from build123d import *
from build123d.topology import SkipClean

# Parameters (mm, degrees)
SKETCH1_W                  = 22
SKETCH1_H                  = 39
SKETCH1_W_2                = 6
SKETCH1_H_2                = 8
BOSS_EXTRUDE1_DEPTH        = 8.25
SKETCH8_W                  = 15.1
SKETCH8_H                  = 11.4
CUT_EXTRUDE3_DEPTH         = 2.25
SKETCH7_R                  = 2.825
SKETCH7_R_2                = 0.825
CUT_EXTRUDE4_DEPTH         = 1.25
SKETCH9_R                  = 0.75
CUT_EXTRUDE5_DEPTH         = 39.274404999
CUT_EXTRUDE1_DEPTH         = 37.440988331
CUT_EXTRUDE1_DEPTH_BACK    = 39.690988331
CUT_EXTRUDE1_START         = 2.25
SKETCH6_R                  = 2.825
BOSS_EXTRUDE2_DEPTH        = 8.25
FILLET3_R                  = 4
FILLET4_R                  = 2
CUT_EXTRUDE7_DEPTH         = 39.900472274
FILLET5_R                  = 7
F_2_2_2_2_DIAMETER_HOLE1_D = 2.2
FILLET6_R                  = 2


with BuildPart() as part:
    # Sketch1 → Boss-Extrude1 (new body)
    with BuildSketch(Plane(origin=(0, 0, 0), x_dir=(1, 0, 0), z_dir=(0, 1, 0))):
        with Locations((21.383330249, 0)):
            Rectangle(SKETCH1_W, SKETCH1_H)
        with Locations((22.383330249, 0)):
            Rectangle(SKETCH1_W_2, SKETCH1_H_2, mode=Mode.SUBTRACT)
    extrude(amount=BOSS_EXTRUDE1_DEPTH)

    # Sketch8 → Cut-Extrude3 (cut)
    with BuildSketch(Plane(origin=(0, 8.25, 0), x_dir=(1, 0, 0), z_dir=(0, 1, 0))):
        with Locations((23.333330249, -12)):
            Rectangle(SKETCH8_W, SKETCH8_H)
        with Locations((23.333330249, 12)):
            Rectangle(SKETCH8_W, SKETCH8_H)
    extrude(amount=-CUT_EXTRUDE3_DEPTH, mode=Mode.SUBTRACT)

    # Sketch7 → Cut-Extrude4 (cut)
    with BuildSketch(Plane(origin=(0, 6, 0), x_dir=(1, 0, 0), z_dir=(0, 1, 0))):
        with Locations(Location((24.633330249, 12, 0), (0, 0, 270))):
            Circle(SKETCH7_R)
        with Locations(Location((20.140330249, 14.5, 0), (0, 0, 270))):
            Circle(SKETCH7_R_2)
        with Locations(Location((27.633330249, 14.5, 0), (0, 0, 270))):
            Circle(SKETCH7_R_2)
        with Locations(Location((27.633330249, 9.5, 0), (0, 0, 270))):
            Circle(SKETCH7_R_2)
        with Locations(Location((20.140330249, 9.5, 0), (0, 0, 270))):
            Circle(SKETCH7_R_2)
        with Locations(Location((20.140330249, -9.5, 0), (0, 0, 90))):
            Circle(SKETCH7_R_2)
        with Locations(Location((27.633330249, -9.5, 0), (0, 0, 90))):
            Circle(SKETCH7_R_2)
        with Locations(Location((27.633330249, -14.5, 0), (0, 0, 90))):
            Circle(SKETCH7_R_2)
        with Locations(Location((20.140330249, -14.5, 0), (0, 0, 90))):
            Circle(SKETCH7_R_2)
        with Locations(Location((24.633330249, -12, 0), (0, 0, 90))):
            Circle(SKETCH7_R)
    extrude(amount=-CUT_EXTRUDE4_DEPTH, mode=Mode.SUBTRACT)

    # Sketch9 → Cut-Extrude5 (cut, through all)
    with BuildSketch(Plane(origin=(0, 6, 0), x_dir=(1, 0, 0), z_dir=(0, 1, 0))):
        with Locations(Location((17.633330249, 14.5, 0), (0, 0, 270))):
            Circle(SKETCH9_R)
        with Locations(Location((17.633330249, 12, 0), (0, 0, 270))):
            Circle(SKETCH9_R)
        with Locations(Location((17.633330249, 9.5, 0), (0, 0, 270))):
            Circle(SKETCH9_R)
        with Locations(Location((30.133330249, 12, 0), (0, 0, 270))):
            Circle(SKETCH9_R)
        with Locations((30.133330249, -12)):
            Circle(SKETCH9_R)
        with Locations(Location((17.633330249, -9.5, 0), (0, 0, 90))):
            Circle(SKETCH9_R)
        with Locations(Location((17.633330249, -12, 0), (0, 0, 90))):
            Circle(SKETCH9_R)
        with Locations(Location((17.633330249, -14.5, 0), (0, 0, 90))):
            Circle(SKETCH9_R)
    extrude(amount=-CUT_EXTRUDE5_DEPTH, mode=Mode.SUBTRACT)

    # Sketch6 → Cut-Extrude1 (cut, two sides: drawn at the far end of the back side and taken through both)
    with BuildSketch(Plane(origin=(0, 8.25, 0), x_dir=(-1, 0, 0), z_dir=(0, -1, 0)).offset(CUT_EXTRUDE1_START - CUT_EXTRUDE1_DEPTH_BACK)):
        with Locations((-24.633330249, -12)):
            Circle(SKETCH6_R)
        with Locations((-24.633330249, 12)):
            Circle(SKETCH6_R)
        Polygon((-26.045830249, -9.553478234), (-25.720830249, -10.116394747), (-12.730449192, -2.616394747), (-13.055449192, -2.053478234), align=None)
        Polygon((-13.055449192, 2.053478234), (-12.730449192, 2.616394747), (-25.720830249, 10.116394747), (-26.045830249, 9.553478234), align=None)
    extrude(amount=CUT_EXTRUDE1_DEPTH + CUT_EXTRUDE1_DEPTH_BACK, mode=Mode.SUBTRACT)

    # Sketch11 → Boss-Extrude2 (add, through all)
    with BuildSketch(Plane(origin=(0, 8.25, 0), x_dir=(1, 0, 0), z_dir=(0, 1, 0))):
        with BuildLine():
            ThreePointArc((32.383330249, 10.801042119), (32.633330249, 12), (32.383330249, 13.198957881))
            Line((32.383330249, 13.198957881), (32.383330249, 10.801042119))
        make_face()
        with BuildLine():
            ThreePointArc((32.383330249, -13.198957881), (32.633330249, -12), (32.383330249, -10.801042119))
            Line((32.383330249, -10.801042119), (32.383330249, -13.198957881))
        make_face()
    extrude(amount=-BOSS_EXTRUDE2_DEPTH)

    # Fillet3
    fillet3_edges = [part.edges().sort_by_distance(p)[0] for p in [
        (30.883330249, 7.125, -17.7),
        (30.883330249, 7.125, -6.3),
        (30.883330249, 7.125, 6.3),
        (30.883330249, 7.125, 17.7),
    ]]
    fillet(fillet3_edges, radius=FILLET3_R)

    # Fillet4
    fillet4_edges = [part.edges().sort_by_distance(p)[0] for p in [
        (25.383330249, 4.125, -4),
        (19.383330249, 4.125, -4),
        (19.383330249, 4.125, 4),
        (25.383330249, 4.125, 4),
    ]]
    fillet(fillet4_edges, radius=FILLET4_R)

    # Sketch11<4> → Cut-Extrude7 (cut, through all)
    with SkipClean():  # the faces are left unmerged after this step: merging them gives an invalid solid
        with BuildSketch(Plane(origin=(0, 8.25, 0), x_dir=(1, 0, 0), z_dir=(0, 1, 0))):
            with BuildLine():
                Line((28.767304845, 19.5), (29.633330249, 18))
                Line((29.633330249, 18), (29.80653533, 17.7))
                Line((29.80653533, 17.7), (30.883330249, 17.7))
                Line((30.883330249, 17.7), (30.883330249, 15.834936491))
                Line((30.883330249, 15.834936491), (32.231406461, 13.5))
                ThreePointArc((32.231406461, 13.5), (32.311601404, 13.351615189), (32.383330249, 13.198957881))
                Line((32.383330249, 13.198957881), (32.383330249, 19.5))
                Line((32.383330249, 19.5), (28.767304845, 19.5))
            make_face()
            Polygon((30.883330249, 17.7), (29.80653533, 17.7), (30.883330249, 15.834936491), align=None)
            with BuildLine():
                Line((32.383330249, -10.801042119), (32.383330249, 10.801042119))
                ThreePointArc((32.383330249, 10.801042119), (32.311601404, 10.648384811), (32.231406461, 10.5))
                Line((32.231406461, 10.5), (30.883330249, 8.165063509))
                Line((30.883330249, 8.165063509), (30.883330249, 6.3))
                Line((30.883330249, 6.3), (29.80653533, 6.3))
                Line((29.80653533, 6.3), (29.633330249, 6))
                Line((29.633330249, 6), (29.633330249, -6))
                Line((29.633330249, -6), (29.80653533, -6.3))
                Line((29.80653533, -6.3), (30.883330249, -6.3))
                Line((30.883330249, -6.3), (30.883330249, -8.165063509))
                Line((30.883330249, -8.165063509), (32.231406461, -10.5))
                ThreePointArc((32.231406461, -10.5), (32.311601404, -10.648384811), (32.383330249, -10.801042119))
            make_face()
            Polygon((30.883330249, 6.3), (30.883330249, 8.165063509), (29.80653533, 6.3), align=None)
            with BuildLine():
                Line((32.383330249, -19.5), (32.383330249, -13.198957881))
                ThreePointArc((32.383330249, -13.198957881), (32.311601404, -13.351615189), (32.231406461, -13.5))
                Line((32.231406461, -13.5), (30.883330249, -15.834936491))
                Line((30.883330249, -15.834936491), (30.883330249, -17.7))
                Line((30.883330249, -17.7), (29.80653533, -17.7))
                Line((29.80653533, -17.7), (29.633330249, -18))
                Line((29.633330249, -18), (28.767304845, -19.5))
                Line((28.767304845, -19.5), (32.383330249, -19.5))
            make_face()
            Polygon((30.883330249, -17.7), (30.883330249, -15.834936491), (29.80653533, -17.7), align=None)
            Polygon((29.80653533, -6.3), (30.883330249, -8.165063509), (30.883330249, -6.3), align=None)
        extrude(amount=-CUT_EXTRUDE7_DEPTH, mode=Mode.SUBTRACT)

    # Fillet5
    fillet5_edges = [part.edges().sort_by_distance(p)[0] for p in [
        (10.383330249, 4.125, 19.5),
        (10.383330249, 4.125, -19.5),
    ]]
    fillet(fillet5_edges, radius=FILLET5_R)

    # Ø2.2 (2.2) Diameter Hole1 (through all)
    with Locations(Plane(origin=(12.883330249, 8.25, -12), x_dir=(0, 0, 1), z_dir=(0, 1, 0))):
        with Locations((0, 0), (12, 14.5), (24, 0)):
            Hole(F_2_2_2_2_DIAMETER_HOLE1_D / 2)

    # Fillet6
    fillet6_edges = [part.edges().sort_by_distance(p)[0] for p in [
        (28.767304845, 4.125, -19.5),
        (28.767304845, 4.125, 19.5),
    ]]
    fillet(fillet6_edges, radius=FILLET6_R)


solid = part.part
CAD build for the part. Positions are in the model's coordinates, mm. A direction names the side the tool comes from. Round coordinates to 2 decimals unless told otherwise and drop trailing zeros. Order: outer loops, then holes, each group sorted by start corner. A loop starts at its lowest first (then second) coordinate and runs counter-clockwise, first axis right, second up. Notation, with made-up numbers: (4, 62) - (45, 62) arc R19 ccw to (45, 87) - close; hole circle Ø4 at (-10.5, 47.25). An arc over 180 degrees is marked (long way). Return JSON: item names as keys, results as strings.
(1) Cut at A-A (z = -3.5). Give the cut face in (x, y).
Answer key:
{"outline": "(10.38, 0) - (14.26, 0) - (14.26, 8.25) - (10.38, 8.25) - close; (15.56, 0) - (20.06, 0) - (20.06, 8.25) - (15.56, 8.25) - close; (24.71, 0) - (29.63, 0) - (29.63, 8.25) - (24.71, 8.25) - close"}
(2) Pin check, flat tips, straight feed: pin 1 Ø1.5 at (x, y) = (12.5, 1) entering from -Z; pin 2 Ø12 at (x, z) = (13, 10.5) entering from -Y; pin 3 Ø2 at (x, y) = (30, 1.5) entering from +Z; pin 4 Ø4.5 at (y, z) = (4, 0) entering from +X. Stop position of each tip, or through.
Answer key:
{"pin 1": "stops at z = -18.15", "pin 2": "stops at y = 0", "pin 3": "stops at z = 18.94", "pin 4": "stops at x = 29.63"}
(3) Cut at B-B (x = 31.25). Give the cut face in (y, z).
Answer key:
{"outline": "(0, -15.2) - (8.25, -15.2) - (8.25, -8.8) - (0, -8.8) - close; (0, 8.8) - (8.25, 8.8) - (8.25, 15.2) - (0, 15.2) - close"}
(4) Wall check: probe 1 along X at (y, z) = (5.25, 12); probe 2 along Z at (x, y) = (27.75, 7); probe 3 along X at (y, z) = (5.45, 14.5). Give the ranges that are in metal, low to high. Write a range as from..to.
Answer key:
{"probe 1": "x = 10.38..11.78, 13.98..16.88, 18.38..21.81, 27.46..29.38, 30.88..32.63", "probe 2": "z = -19.5..-17.6, -6.4..-1.04, 1.04..6.4, 17.6..19.5", "probe 3": "x = 10.68..16.88, 18.38..19.32, 20.97..23.32, 25.95..26.81, 28.46..31.65"}
(5) Tool access for faces 5 (the face through (20, 4.75, -10)), 6 (the face through (22, 4, -4)), 7 (the face through (12.379, 4.183, -17.395)): list every direction of +Z, -Z, +X, -X, +Y, -Y with a clear straight run to the whole face (end or side of a thin tool).
Answer key:
{"face 5": "+Y", "face 6": "+Y, -Y", "face 7": "-Z, -X, +Y, -Y"}
(6) Pull direction X, two halves, no side cores. Call faces 1 (the face through (29.633, 4, 0)), 2 (the face through (18.14, 3.042, -10.053)), 3 (the face through (10.383, 4, 0)), 4 (the face through (19.583, 5.384, 10.108)): +X half, -X half, draft (parallel to the pull), parting line (faces both ways), or undercut.
Answer key:
{"face 1": "+X half", "face 2": "undercut", "face 3": "-X half", "face 4": "undercut"}
(7) Cut at C-C (y = 5.5). State how many separate pieces and enclosed holes the cut face has, then the cut area to 3 significant figures.
Answer key:
{"separate pieces": "1", "enclosed holes": "22", "area": "613 mm^2"}
